Solid Edge part; units mm, degrees
sketch "Sketch1" plane through (0, 0, 0) normal (0, 0, 1) x (1, 0, 0)
  line L0 (48.4569, -123.3254) -> (-7.5, -3.3254)
  line L1 (-7.5, -3.3254) -> (-7.5, 106.6746)
  line L2 (-7.5, 106.6746) -> (7.5, 106.6746)
  line L3 (7.5, 106.6746) -> (7.5, 0)
  line L4 (7.5, 0) -> (62.0515, -116.9861)
  line L5 (62.0515, -116.9861) -> (48.4569, -123.3254)
extrude "Protrusion1" add sketch "Sketch1" along normal blind 3
sketch "Sketch2" plane through (33.3013, -25.359, 3) normal (0, 0, 1) x (0, -1, 0)
  line L0 (121.5304, 26.1437) -> (119.84, 29.769)
  line L1 (119.84, 29.769) -> (96.276, 18.7809)
  line L2 (96.276, 18.7809) -> (97.9664, 15.1556)
  line L3 (97.9664, 15.1556) -> (121.5304, 26.1437)
extrude "Protrusion2" add sketch "Sketch2" against normal up to surface (3 mm away)
sketch "Sketch3" plane through (35.3731, -35.2776, 3) normal (0, 0, 1) x (0, -1, 0)
  circle A0 centre (-33.6149, -35.3731) radius 2.5
extrude "Cutout1" cut sketch "Sketch3" against normal up to next
fillet "Arrondis_angles" radius 2 2 edges at (-7.5, -3.3254, 1.5) (7.5, 0, 1.5)
fillet "Arrondis_0" radius 0.5 8 edges at (26.0662, -75.3083, 0) (26.0662, -75.3083, 3) (34.8695, -58.694, 0) (34.8695, -58.694, 3) (-7.5, 51.8963, 3) (7.5, 53.559, 3) (7.5, 53.559, 0) (-7.5, 51.8963, 0)
Input: part model. Units: mm. Frame: model coordinates. A direction names the side the tool comes from. Coordinates: 2 decimals unless noted, no trailing zeros. Loops run counter-clockwise (first coordinate to the right, second up) from the corner with the lowest first, then second, coordinate; pieces in that order, holes last.
Q1. Set-up query: faces 1 (the flat face through (57.653, -133.582, 1.521)), 2 (the cylindrical face through (35.11, -59.57, 0.14)). Return all of +Z, -Z, +X, -X, +Y, -Y with unobstructed straight access to the full face (end or side cutting, diameter ignored); none if empty.
Results are:
face 1: +Z, -Z, +X
face 2: -Z, +X, +Y
Q2. Section A-A, the plane z = 1.15. Return the cut outline in (x, y) (1 decimal), and give its area (3 significant figures).
Results are:
outline: (-7.5, -2.9) arc R2 ccw to (-7.3, -3.7) - (48.5, -123.3) - (59.4, -146.9) - (63.1, -145.2) - (52.1, -121.6) - (62.1, -117) - (7.7, -0.4) arc R2 cw to (7.5, 0.4) - (7.5, 106.7) - (-7.5, 106.7) - close; hole circle Ø5 at (0, -1.7)
area: 3,670 mm2
Q3. Line query: line 1 along X through (y, z) = (17, 0.85); line 2 along Y through (x, z) = (57.5, 1.55); line 3 along Y through (x, z) = (-1, 1.1). Output: solid intervals per line, ascending.
Results are:
line 1: x = -7.5 to 7.5
line 2: y = -142.72 to -133.25, -119.11 to -107.23
line 3: y = -17.26 to -3.95, 0.63 to 106.67
Q4. Contact query for a flat-ended pin moving along its axis: pin 1 (1 mm diameter, centred on y = 77.5, z = 1.5, fed in from +X). Output: stop coordinate, or through.
Results are:
pin 1: stops at x = 7.5
Q5. Mould query, pull axis X, two halves, no side actions, for faces 3 (the cylindrical face through (35.12, -59.57, 2.85)), 4 (the flat face through (15, -19, 3)), 5 (the cylindrical face through (-1.52, 0.32, 1.52)). Classes: +X half, -X half, draft (parallel to the pull), parting line (faces both ways), or undercut.
Results are:
face 3: +X half
face 4: draft
face 5: undercut
